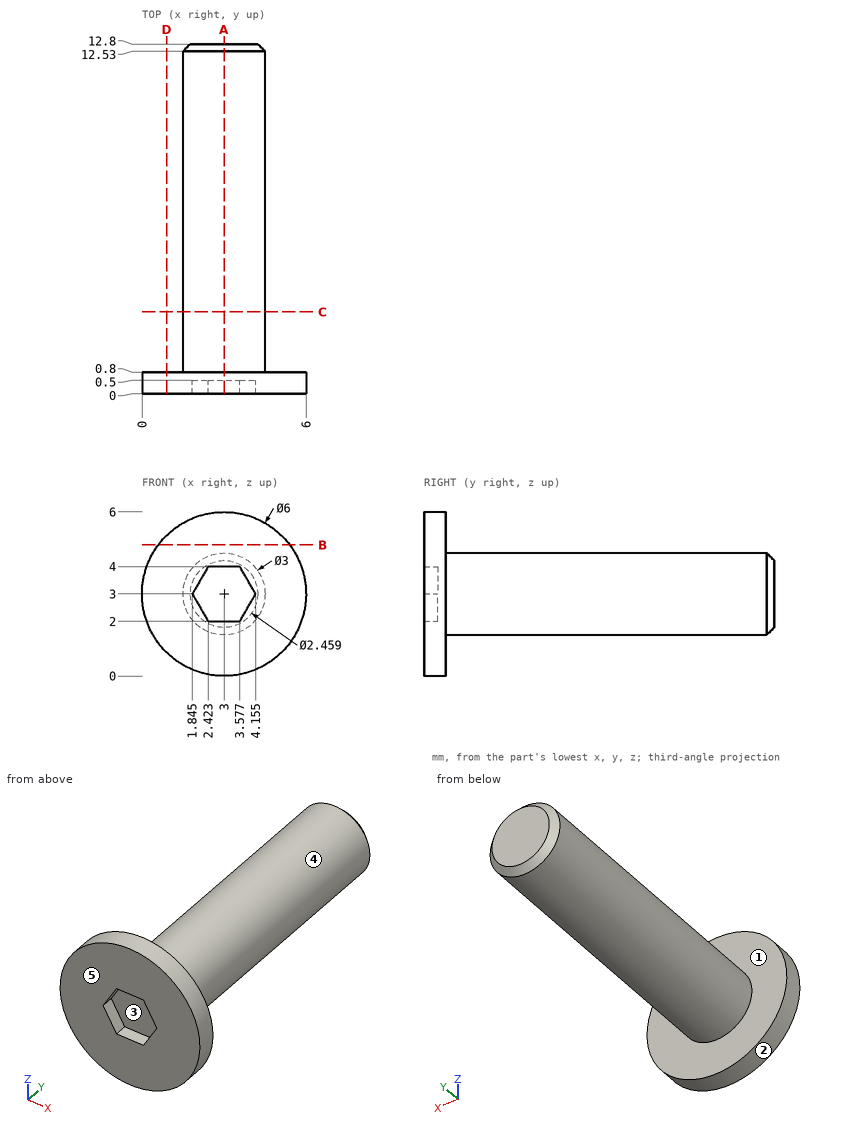
Could you check a few things on this drawing? It's one solid part, dimensions in mm from its lowest x, y, z. A direction names the side the tool comes from. Round coordinates to 2 decimals unless told otherwise and drop trailing zeros. Order: outer loops, then holes, each group sorted by start corner. A loop starts at its lowest first (then second) coordinate and runs counter-clockwise, first axis right, second up.
Q1. I'm going to push flat-ended pins straight in: P1, Ø0.6, axis at x = 3.5, z = 3, coming from the -Y side; P2, Ø1.5, axis at x = 3, y = 4.5, coming from the -Z side. Where does each tip first touch, or does it pass through?
Geometry says:
P1: stops at y = 0.5
P2: stops at z = 1.5
Q2. Imagine slicing it at D-D, the plane x = 0.9. List the corners of the cut face in (y, z) for me.
Geometry says:
outline: (0, 0.86) - (0.8, 0.86) - (0.8, 5.14) - (0, 5.14) - close
Q3. Please list where these lines run through material, in increasing order: probe 1 along Y at (x, z) = (2.6, 5.75); probe 2 along Y at (x, z) = (2.25, 3.4); probe 3 along X at (y, z) = (3.5, 2.65).
Geometry says:
probe 1: y = 0 to 0.8
probe 2: y = 0.5 to 12.8
probe 3: x = 1.54 to 4.46
Q4. Imagine slicing it at B-B, the plane z = 4.8. List the corners of the cut face in (x, y) for me.
Geometry says:
outline: (0.6, 0) - (5.4, 0) - (5.4, 0.8) - (0.6, 0.8) - close
Q5. Imagine slicing it at C-C, the plane y = 3. List the corners of the cut face in (x, z) for me.
Geometry says:
outline: circle Ø3 at (3, 3)
Q6. Which directions (+Z, -Z, +X, -X, +Y, -Y) give clear straight access to the entire face, cutting with the end or side of a thin tool? Please do the marked faces 4 and 5.
Geometry says:
face 4: +Y
face 5: +Z, -Z, +X, -X, -Y
Q7. Imagine slicing it at A-A, the plane x = 3. List the corners of the cut face in (y, z) for me.
Geometry says:
outline: (0, 0) - (0.8, 0) - (0.8, 1.5) - (12.53, 1.5) - (12.8, 1.77) - (12.8, 4.23) - (12.53, 4.5) - (0.8, 4.5) - (0.8, 6) - (0, 6) - (0, 4) - (0.5, 4) - (0.5, 2) - (0, 2) - close
Q8. Thinking about a two-plate mould opening in X: for the marked faces 1, 2 and 3, which applies, released by +X, released by -X, zero draft, split by the parting line, or undercut?
Geometry says:
face 1: zero draft
face 2: split by the parting line
face 3: undercut
